Read the model definition and answer for the solid it produces. Units are mm, in the model's axes. Face numbers are marked on the shaded views. Give positions to 0.01 mm unless a question says otherwise; leave off trailing zeros. Write each loop counter-clockwise with the first axis right and the second up, starting at its lowest first coordinate (ties: lowest second). Pieces come first, ordered by that corner, then holes. Notation, with made-up numbers: (10.25, 9.25) -> (42.25, 9.25) arc R21 cw to (42.25, 30.25) -> close; hole circle Ø1 at (-4, 29.25). An arc over 180 degrees is marked (long way). Use a Markdown table: item, result.
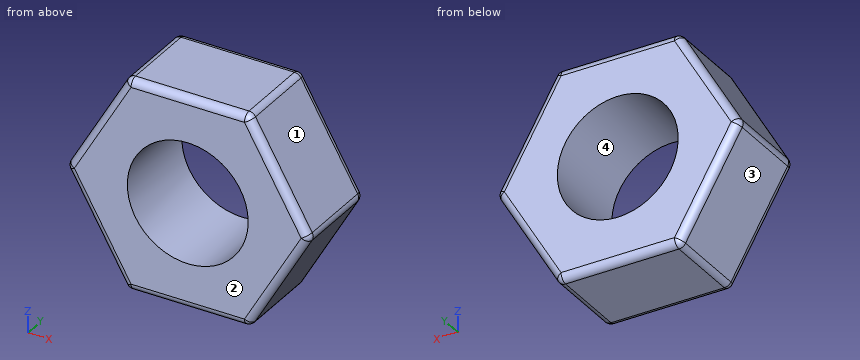
from build123d import *

# Parameters (mm, degrees)
SKETCH1_R           = 2
BOSS_EXTRUDE1_DEPTH = 3
FILLET1_R           = 0.25


with BuildPart() as part:
    # Sketch1 → Boss-Extrude1 (new body)
    with BuildSketch(Plane(origin=(0, 0, 0), x_dir=(1, 0, 0), z_dir=(0, 1, 0))):
        Polygon((-2.020725942, 3.5), (-4.041451884, 0), (-2.020725942, -3.5), (2.020725942, -3.5), (4.041451884, 0), (2.020725942, 3.5), align=None)
        Circle(SKETCH1_R, mode=Mode.SUBTRACT)
    extrude(amount=BOSS_EXTRUDE1_DEPTH)

    # Fillet1
    fillet1_edges = [part.edges().sort_by_distance(p)[0] for p in [
        (2.020725942, 1.5, -3.5),
        (4.041451884, 1.5, 0),
        (2.020725942, 1.5, 3.5),
        (-2.020725942, 1.5, 3.5),
        (-4.041451884, 1.5, 0),
        (-2.020725942, 1.5, -3.5),
        (-3.031088913, 3, 1.75),
        (0, 3, 3.5),
        (3.031088913, 3, 1.75),
        (3.031088913, 3, -1.75),
        (0, 3, -3.5),
        (3.031088913, 0, -1.75),
        (3.031088913, 0, 1.75),
        (0, 0, 3.5),
        (-3.031088913, 0, 1.75),
        (-3.031088913, 0, -1.75),
        (0, 0, -3.5),
        (-3.031088913, 3, -1.75),
    ]]
    fillet(fillet1_edges, radius=FILLET1_R)


solid = part.part
Item 1: A cutting plane is placed at A-A (x = 0). Give the vertices of the cut face in (y, z).
Return value:
| item | result |
|---|---|
| outline | (0, -3.25) arc R0.25 ccw to (0.25, -3.5) -> (2.75, -3.5) arc R0.25 ccw to (3, -3.25) -> (3, -2) -> (0, -2) -> close; (0, 2) -> (3, 2) -> (3, 3.25) arc R0.25 ccw to (2.75, 3.5) -> (0.25, 3.5) arc R0.25 ccw to (0, 3.25) -> close |
Item 2: For a pull along Z with two mould halves and no side action, classify the marked faces 1, 2, 3 and 4 as +Z half, -Z half, draft (parallel to the pull), parting line (faces both ways), or undercut.
Return value:
| item | result |
|---|---|
| face 1 | +Z half |
| face 2 | draft |
| face 3 | -Z half |
| face 4 | undercut |
Item 3: A cutting plane is placed at B-B (y = 2.5). Give the vertices of the cut face in (x, z) (3 decimals), then the cut area to 3 significant figures.
Return value:
| item | result |
|---|---|
| outline | (-3.969, -0.125) -> (-2.093, -3.375) arc R0.25 ccw to (-1.876, -3.5) -> (1.876, -3.5) arc R0.25 ccw to (2.093, -3.375) -> (3.969, -0.125) arc R0.25 ccw to (3.969, 0.125) -> (2.093, 3.375) arc R0.25 ccw to (1.876, 3.5) -> (-1.876, 3.5) arc R0.25 ccw to (-2.093, 3.375) -> (-3.969, 0.125) arc R0.25 ccw to start; hole circle Ø4 at (0, 0) |
| area | 29.8 mm^2 |
Item 4: A cutting plane is placed at C-C (x = 1.25). Give the vertices of the cut face in (y, z), then the cut area to 3 significant figures.
Return value:
| item | result |
|---|---|
| outline | (0, -3.25) arc R0.25 ccw to (0.25, -3.5) -> (2.75, -3.5) arc R0.25 ccw to (3, -3.25) -> (3, -1.56) -> (0, -1.56) -> close; (0, 1.56) -> (3, 1.56) -> (3, 3.25) arc R0.25 ccw to (2.75, 3.5) -> (0.25, 3.5) arc R0.25 ccw to (0, 3.25) -> close |
| area | 11.6 mm^2 |
Item 5: Straight lines are drawn through the part: line 1 along X through (y, z) = (1.6, 0); line 2 along Z through (x, y) = (0, 1); line 3 along X through (y, z) = (2.85, 1.5). For each, find the intervals that lie inside material, in ascending order. Write a range as [from, to].
Return value:
| item | result |
|---|---|
| line 1 | [-4, -2], [2, 4] |
| line 2 | [-3.5, -2], [2, 3.5] |
| line 3 | [-3.15, -1.32], [1.32, 3.15] |
